from build123d import *

# Parameters (mm, degrees)
F0_R     = 2.38125
F0_R_2   = 1.75
F1_DEPTH = 2.38125
F2_W     = 57.15
F2_H     = 0.79375
F3_DEPTH = 12.5
F5_D     = 1.6
F6_R     = 1


with BuildPart() as f1:
    # F0 (on Front) → F1 (new body, symmetric)
    with BuildSketch(Plane.XZ):
        with BuildLine():
            Line((6.35, -2.38125), (57.575369343, -1.5875))
            ThreePointArc((57.575369343, -1.5875), (63.5, 0), (57.575369343, 1.5875))
            Line((57.575369343, 1.5875), (6.35, 2.38125))
            Line((6.35, 2.38125), (6.35, 6.35))
            Line((6.35, 6.35), (-6.35, 6.35))
            Line((-6.35, 6.35), (-6.35, -6.35))
            Line((-6.35, -6.35), (6.35, -6.35))
            Line((6.35, -6.35), (6.35, -2.38125))
        make_face()
        Circle(F0_R, mode=Mode.SUBTRACT)
        with Locations((60.325, 0)):
            Circle(F0_R_2, mode=Mode.SUBTRACT)
    extrude(amount=F1_DEPTH, both=True)

    # F2 (on Top) → F3 (cut, symmetric)
    with BuildSketch(Plane.XY):
        with Locations((34.925, 1.984375)):
            Rectangle(F2_W, F2_H)
        with Locations((34.925, -1.984375)):
            Rectangle(F2_W, F2_H)
    extrude(amount=F3_DEPTH, both=True, mode=Mode.SUBTRACT)

    # F5 (through all)
    with Locations(Plane(origin=(-6.35, 0, 0), x_dir=(0, -1, 0), z_dir=(-1, 0, 0))):
        with Locations((0, 4.7625), (0, -4.7625)):
            Hole(F5_D / 2)

    # F6
    f6_edges = [f1.edges().sort_by_distance(p)[0] for p in [
        (6.35, 0, 2.38125),
        (6.35, 0, -2.38125),
        (57.575369, 0, 1.5875),
        (57.575369, 0, -1.5875),
    ]]
    fillet(f6_edges, radius=F6_R)


solid = f1.part
Geometry: final body of the model. Coordinates: model frame, mm. A direction names the side the tool comes from. Coordinates: 2 decimals unless noted, no trailing zeros. Write each loop counter-clockwise with the first axis right and the second up, starting at its lowest first coordinate (ties: lowest second). Pieces come first, ordered by that corner, then holes. Notation, with made-up numbers: (88, 21) - (105, 21) arc R24 ccw to (105, 52) - close; hole circle Ø2 at (-5.5, -35). An arc over 180 degrees is marked (long way). Return JSON: item names as keys, results as strings.
Item 1: Section query D-D (x = 18.5). Output: boundary loops of the cut face in (y, z), and give its area (3 significant figures).
Completed:
{"outline": "(-1.59, -2.19) - (1.59, -2.19) - (1.59, 2.19) - (-1.59, 2.19) - close", "area": "13.9 mm2"}
Item 2: Line query: L1, parallel to Z at x = 46.5, y = 1.2; L2, parallel to X at y = 1.05, z = 0.25; L3, parallel to Z at x = 60.5, y = -0.7. Output: solid intervals per line, ascending.
Completed:
{"L1": "z = -1.76 to 1.76", "L2": "x = -6.35 to -2.37, 2.37 to 58.59, 62.06 to 63.49", "L3": "z = -3.17 to -1.74, 1.74 to 3.17"}
Item 3: Reachability of faces 5 (the face through (35, 1.588, 0)), 6 (the face through (35, -1.588, 0)), 7 (the face through (0, 0, 6.35)) from +Z, -Z, +X, -X, +Y, -Y: full face, straight path, thin tool, end or side. Return the list, or none.
Completed:
{"face 5": "+Z, -Z, +X, +Y", "face 6": "+Z, -Z, +X, -Y", "face 7": "+Z, +X, -X, +Y, -Y"}
Item 4: Pull-direction query (Z, two-part tool) for faces 1 (the face through (-1.89, 0.03, -1.45)), 2 (the face through (63.5, 0, -0.1)), 3 (the face through (-6.35, 0, 0)), 4 (the face through (58.577, 0.022, 0.077)); classes: +Z half, -Z half, draft (parallel to the pull), parting line (faces both ways), or undercut.
Completed:
{"face 1": "undercut", "face 2": "parting line", "face 3": "draft", "face 4": "undercut"}
Item 5: Section query A-A (y = 0). Count the separate pieces of the cut face and the enclosed holes in it, and give its area (3 significant figures).
Completed:
{"separate pieces": "3", "enclosed holes": "2", "area": "328 mm2"}
Item 6: Section query B-B (x = 0). Output: boundary loops of the cut face in (y, z).
Completed:
{"outline": "(-2.38, -6.35) - (2.38, -6.35) - (2.38, -2.38) - (-2.38, -2.38) - close; (-2.38, 2.38) - (2.38, 2.38) - (2.38, 6.35) - (-2.38, 6.35) - close; hole circle Ø1.6 at (0, -4.76); hole circle Ø1.6 at (0, 4.76)"}
Item 7: Pin query (flat end, axial travel): pin 1 Ø1 at (x, y) = (16, -1.5) entering from -Z; pin 2 Ø7.5 at (x, z) = (49, 1.5) entering from +Y; pin 3 Ø5.5 at (x, z) = (44, 0) entering from -Y. Return the tip coordinate at first contact, or that it passes through.
Completed:
{"pin 1": "stops at z = -2.24", "pin 2": "stops at y = 1.59", "pin 3": "stops at y = -1.59"}
